Source: CAD feature listing. Evaluate the final solid. Frame: model axes, mm. Give positions to 0.01 mm unless a question says otherwise; leave off trailing zeros. Order: outer loops, then holes, each group sorted by start corner. A loop starts at its lowest first (then second) coordinate and runs counter-clockwise, first axis right, second up.
1) Section C-C, the plane x = -0.5. Return loops of the section in (y, z).
2) Section A-A, the plane y = 0. Return loops of the section in (x, z).
3) Material intervals for line 1 (X direction, y = -1, z = 0.1); line 2 (X direction, y = 2.25, z = 0.3); line 3 (Y direction, x = 3.75, z = 1), sorted ascending.
4) First-contact query: P1, Ø6, axis at x = 2, y = 1.5, coming from the -Z side; P2, Ø2, axis at x = -2, y = -2, coming from the +Z side. Flat tips, straight axial feed; report the tip coordinate or a pass-through.
5) Section B-B, the plane z = 1.3. Return loops of the section in (x, y).
6) Draft query along Y for faces 1 (the face through (2.68, -2.8, 0.52)), 2 (the face through (-0.085, -3.907, 0.733)), 3 (the face through (-0.085, 3.976, 0.764)). Return one class per face: released by +Y, released by -Y, zero draft, split by the parting line, or undercut.
7) Section D-D, the plane z = 0.3. Return loops of the section in (x, y).
Solid Edge part; units mm, degrees
sketch "Sketch1" plane through (0, 0, 0) normal (0, 0, 1) x (1, 0, 0)
  circle A0 centre (0, 0) radius 3.3655
  circle A1 centre (0, 0) radius 6.223
extrude "Protrusion1" add sketch "Sketch1" along normal blind 2.3114
sketch "Sketch2" plane through (0, 0, 0) normal (1, 0, 0) x (0, 1, 0)
  arc A0 (-6.0761, 2.3114) -> (6.0761, 2.3114) centre (0, 9.5328) ccw
  line L0 (-6.0761, 2.3114) -> (6.0761, 2.3114)
  arc A1 (-6.223, 2.1861) -> (-1.351, 0) centre (0, 9.5328) ccw
  line L1 (-1.351, 0) -> (-6.223, 0)
  line L2 (-6.223, 2.1861) -> (-6.223, 0)
  line L3 (6.223, 0) -> (1.351, 0)
  arc A2 (1.351, 0) -> (6.223, 2.1861) centre (0, 9.5328) ccw
  line L4 (6.223, 0) -> (6.223, 2.1861)
extrude "ExtrudedCutout_1" cut sketch "Sketch2" along normal mid plane 38.1
From the geometry:
1. outline: (-6.2, 2.17) arc R9.63 ccw to (-3.33, 0.5) - (-3.33, 0.7) arc R9.44 cw to (-6.08, 2.31) - (-6.2, 2.31) - close; (3.33, 0.5) arc R9.63 ccw to (6.2, 2.17) - (6.2, 2.31) - (6.08, 2.31) arc R9.44 cw to (3.33, 0.7) - close
2. outline: (-6.22, 0) - (-3.37, 0) - (-3.37, 0.1) - (-6.22, 0.1) - close; (3.37, 0) - (6.22, 0) - (6.22, 0.1) - (3.37, 0.1) - close
3. line 1: x = -6.14 to -3.21, 3.21 to 6.14
3. line 2: x = -5.8 to -2.5, 2.5 to 5.8
3. line 3: y = -4.46 to -4.03, 4.03 to 4.46
4. P1: stops at z = 0
4. P2: stops at z = 0.58
5. outline: (-4.18, -4.61) arc R6.22 ccw to (-3.72, -4.99) - (3.72, -4.99) arc R6.22 ccw to (4.18, -4.61) - close; (-4.18, 4.61) - (4.18, 4.61) arc R6.22 ccw to (3.72, 4.99) - (-3.72, 4.99) arc R6.22 ccw to start
6. face 1: undercut
6. face 2: released by -Y
6. face 3: released by +Y
7. outline: (-5.91, -1.96) arc R6.22 ccw to (-5.59, -2.73) - (-1.97, -2.73) arc R3.37 cw to (-2.74, -1.96) - close; (-5.91, 1.96) - (-2.74, 1.96) arc R3.37 cw to (-1.97, 2.73) - (-5.59, 2.73) arc R6.22 ccw to start; (1.97, -2.73) - (5.59, -2.73) arc R6.22 ccw to (5.91, -1.96) - (2.74, -1.96) arc R3.37 cw to start; (1.97, 2.73) arc R3.37 cw to (2.74, 1.96) - (5.91, 1.96) arc R6.22 ccw to (5.59, 2.73) - close
